Can you work these out from the model? Positions are in its coordinate system, mm. Face numbers are marked on the shaded views. A direction names the side the tool comes from. Coordinates: 2 decimals unless noted, no trailing zeros. Order: outer loops, then holes, each group sorted by start corner. A loop starts at its lowest first (then second) coordinate and runs counter-clockwise, first axis right, second up. Notation, with made-up numbers: M -4.5,58 L 47.5,58 A23 cw 47.5,75 Z; hole C 50.5,21.5 d7. An arc over 180 degrees is marked long. Answer as a JSON object with one key per item and string values.
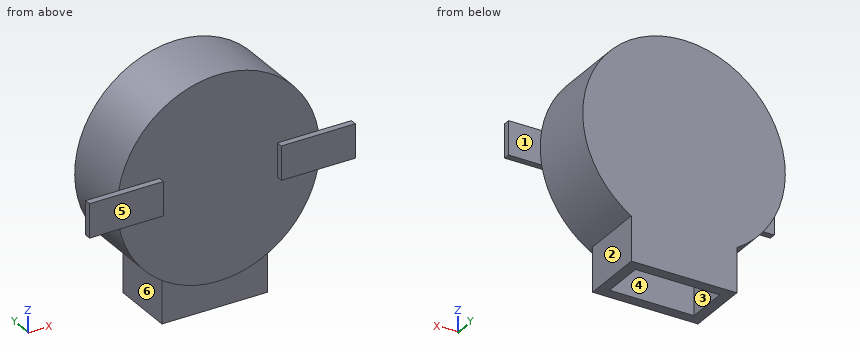
from build123d import *

# Parameters (mm, degrees)
BOSS_EXTRUDE1_DEPTH = 3.3
SKETCH2_W           = 3.5
SKETCH2_H           = 1.6
BOSS_EXTRUDE2_DEPTH = 0.3
CUT_EXTRUDE1_DEPTH  = 0.3
SKETCH4_W           = 4
SKETCH4_H           = 2
CUT_EXTRUDE2_DEPTH  = 3


with BuildPart() as part:
    # Sketch1 → Boss-Extrude1 (new body)
    with BuildSketch(Plane(origin=(0, 0, 0), x_dir=(1, 0, 0), z_dir=(0, 1, 0))):
        with BuildLine():
            Line((-2.5, 4.09756025), (-2.5, 6.2))
            Line((-2.5, 6.2), (2.5, 6.2))
            Line((2.5, 6.2), (2.5, 4.09756025))
            ThreePointArc((2.5, 4.09756025), (0, -4.8), (-2.5, 4.09756025))
        make_face()
    extrude(amount=BOSS_EXTRUDE1_DEPTH)

    # Sketch2 → Boss-Extrude2 (add)
    with BuildSketch(Plane.XZ):
        with Locations((-4.55, 0)):
            Rectangle(SKETCH2_W, SKETCH2_H)
        with Locations((4.55, 0)):
            Rectangle(SKETCH2_W, SKETCH2_H)
    extrude(amount=BOSS_EXTRUDE2_DEPTH)

    # Sketch3 → Cut-Extrude1 (cut)
    with BuildSketch(Plane.XZ):
        with BuildLine():
            Line((2.5, -4.09756025), (2.5, -6.2))
            Line((2.5, -6.2), (-2.5, -6.2))
            Line((-2.5, -6.2), (-2.5, -4.09756025))
            ThreePointArc((-2.5, -4.09756025), (0, -4.8), (2.5, -4.09756025))
        make_face()
    extrude(amount=-CUT_EXTRUDE1_DEPTH, mode=Mode.SUBTRACT)

    # Sketch4 → Cut-Extrude2 (cut)
    with BuildSketch(Plane(origin=(0, 0, -6.2), x_dir=(-1, 0, 0), z_dir=(0, 0, -1))):
        with Locations((0, 1.8)):
            Rectangle(SKETCH4_W, SKETCH4_H)
    extrude(amount=-CUT_EXTRUDE2_DEPTH, mode=Mode.SUBTRACT)


solid = part.part
Item 1: I want a section at C-C, the plane y = 1.05. Write out the boundary of the cut face in (x, z), plus the area to 3 significant figures.
Answers follow:
{"outline": "M -2.5,-6.2 L -2,-6.2 L -2,-3.2 L 2,-3.2 L 2,-6.2 L 2.5,-6.2 L 2.5,-4.1 A4.8 ccw long -2.5,-4.1 Z", "area": "68.5 mm^2"}
Item 2: I'm going to push flat-ended pins straight in: pin 1 (2.5 mm diameter, centred on x = -0.5, z = -5, fed in from -Y); pin 2 (1.7 mm diameter, centred on y = 2.5, z = -5, fed in from -X); pin 3 (0.6 mm diameter, centred on y = 2, z = -4.5, fed in from +X). Where does each tip first touch, or does it pass through?
Answers follow:
{"pin 1": "stops at y = 0", "pin 2": "stops at x = -2.5", "pin 3": "stops at x = 2.5"}
Item 3: I want a section at D-D, the plane z = 0. Write out the boundary of the cut face in (x, y).
Answers follow:
{"outline": "M -6.3,-0.3 L -2.8,-0.3 L -2.8,0 L 2.8,0 L 2.8,-0.3 L 6.3,-0.3 L 6.3,0 L 4.8,0 L 4.8,3.3 L -4.8,3.3 L -4.8,0 L -6.3,0 Z"}
Item 4: I want a section at A-A, the plane z = -5.5. Write out the boundary of the cut face in (x, y).
Answers follow:
{"outline": "M -2.5,0.3 L 2.5,0.3 L 2.5,3.3 L -2.5,3.3 Z; hole M -2,0.8 L 2,0.8 L 2,2.8 L -2,2.8 Z"}
Item 5: If we mould it in two halves opening along X, with no side actions, what happens to the marked faces 1, 2, 3 and 4? For each: pulls with the +X half, pulls with the -X half, needs draft (parallel to the pull), parting line crosses it, or undercut.
Answers follow:
{"face 1": "needs draft", "face 2": "pulls with the +X half", "face 3": "undercut", "face 4": "undercut"}
Item 6: Which directions (+Z, -Z, +X, -X, +Y, -Y) give clear straight access to the entire face, cutting with the end or side of a thin tool? Please do the marked faces 5 and 6.
Answers follow:
{"face 5": "+Z, -Z, +X, -X, -Y", "face 6": "-Z, -X, +Y, -Y"}
Item 7: I want a section at B-B, the plane x = -3.25. Write out the boundary of the cut face in (y, z).
Answers follow:
{"outline": "M -0.3,-0.8 L 0,-0.8 L 0,-3.53 L 3.3,-3.53 L 3.3,3.53 L 0,3.53 L 0,0.8 L -0.3,0.8 Z"}
Item 8: Please list where these lines run through material, in increasing order: line 1 (X direction, y = 0.9, z = -4.75); line 2 (Y direction, x = 1.75, z = -4.75); line 3 (Y direction, x = 0, z = 3.25).
Answers follow:
{"line 1": "x = -2.5 to -2, 2 to 2.5", "line 2": "y = 0.3 to 0.8, 2.8 to 3.3", "line 3": "y = 0 to 3.3"}
